Verification items for the finished model (mm, model axes). A direction names the side the tool comes from. Round coordinates to 2 decimals unless told otherwise and drop trailing zeros. Order: outer loops, then holes, each group sorted by start corner. A loop starts at its lowest first (then second) coordinate and runs counter-clockwise, first axis right, second up. Notation, with made-up numbers: (11.5, -2) -> (24.5, -2) arc R26 cw to (24.5, 24) -> close; hole circle Ø2 at (58, 35). An arc over 180 degrees is marked (long way). Return JSON: item names as keys, results as strings. Group by question number.
1) Scan lines: L1, parallel to Z at x = 7, y = 27; L2, parallel to Y at x = 4, z = 15.5; L3, parallel to Y at x = 14.5, z = 21. Record each from-to range of solid material in increasing order.
2) Section check B-B on x = 6. Enter the section's corners in (y, z).
3) Depth check by flat-ended pin: pin 1 (10 mm diameter, centred on x = 11, y = 4, fed in from -Z); pin 2 (8 mm diameter, centred on x = 25.5, z = 23.5, fed in from -Y); pin 3 (5 mm diameter, centred on y = 8, z = 8.5, fed in from -X); pin 4 (6.5 mm diameter, centred on x = 6.5, z = 42.5, fed in from +Y). Enter the tip coordinate at first touch or a pass-through.
4) Section check A-A on z = 13. Enter the section's corners in (x, y), plus the area to 3 significant figures.
5) Section check C-C on y = 4.5. Enter the section's corners in (x, z).
6) Tool access check on faces 1 (the flat face through (15, -5, 5.691)), 2 (the flat face through (15, 15, 20)), 3 (the flat face through (19.788, -5, 18)), 4 (the flat face through (10.428, -5, 18)). Record the directions out of +Z, -Z, +X, -X, +Y, -Y that give a thin tool (end or side, any length) a straight path to the whole face; none if there is none.
```python
from build123d import *

# Parameters (mm, degrees)
SKETCH1_W           = 30
SKETCH1_H           = 30
BOSS_EXTRUDE1_DEPTH = 20
SKETCH2_W           = 9.360375711
SKETCH2_H           = 14.309479907
BOSS_EXTRUDE2_DEPTH = 10
BOSS_EXTRUDE3_DEPTH = 10


with BuildPart() as part:
    # Sketch1 → Boss-Extrude1 (new body)
    with BuildSketch(Plane.XY):
        with Locations((15, 15)):
            Rectangle(SKETCH1_W, SKETCH1_H)
    extrude(amount=BOSS_EXTRUDE1_DEPTH)

    # Sketch2 → Boss-Extrude2 (add)
    with BuildSketch(Plane.XZ):
        with Locations((15.108123152, 12.845260046)):
            Rectangle(SKETCH2_W, SKETCH2_H)
    extrude(amount=BOSS_EXTRUDE2_DEPTH)

    # Sketch3 → Boss-Extrude3 (add)
    with BuildSketch(Plane.XZ.offset(10)):
        Polygon((10.427935296, 29.980050477), (-2.268076866, 53.225538566), (6.759662186, 58.156228099), (19.788311007, 29.980050477), (19.788311007, 20), (10.427935296, 20), align=None)
    extrude(amount=-BOSS_EXTRUDE3_DEPTH)


solid = part.part
```
Check result:
{
 "1": {"L1": "0 to 20", "L2": "0 to 30", "L3": "-10 to 0"},
 "2": {"outline": "(-10, 38.09) -> (0, 38.09) -> (0, 57.74) -> (-10, 57.74) -> close; (0, 0) -> (30, 0) -> (30, 20) -> (0, 20) -> close"},
 "3": {"pin 1": "z = 0", "pin 2": "y = 0", "pin 3": "x = 0", "pin 4": "y = 0"},
 "4": {"outline": "(0, 0) -> (10.43, 0) -> (10.43, -10) -> (19.79, -10) -> (19.79, 0) -> (30, 0) -> (30, 30) -> (0, 30) -> close", "area": "994 mm^2"},
 "5": {"outline": "(0, 0) -> (30, 0) -> (30, 20) -> (0, 20) -> close"},
 "6": {"face 1": "-Z, +X, -X, -Y", "face 2": "+Z, +X, -X, +Y", "face 3": "+Z, -Z, +X, -Y", "face 4": "-Z, -X, -Y"}
}
